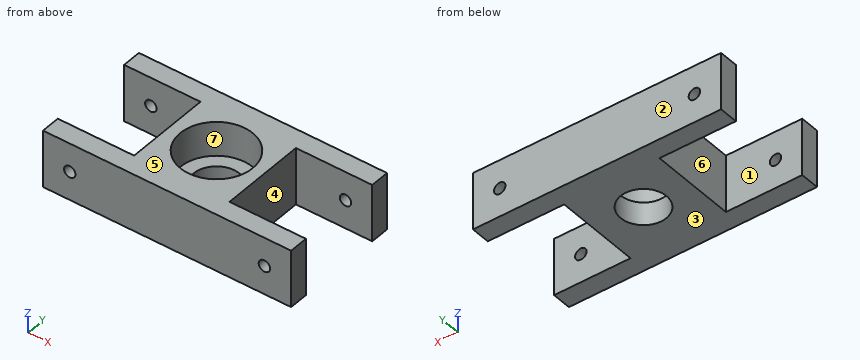
Autodesk Inventor part; units mm, degrees
ref_plane "YZ Plane" through (0, 0, 0) normal (1, 0, 0) x (0, 1, 0)
ref_plane "XZ Plane" through (0, 0, 0) normal (0, 1, 0) x (-1, 0, 0)
ref_plane "XY Plane" through (0, 0, 0) normal (0, 0, 1) x (1, 0, 0)
sketch "Boceto1" plane through (0, 0, 0) normal (0, 0, 1) x (1, 0, 0)
  line L0 (-12.5, 16.25) -> (12.5, 16.25)
  line L1 (12.5, 16.25) -> (12.5, -16.25)
  line L2 (12.5, -16.25) -> (-12.5, -16.25)
  line L3 (-12.5, -16.25) -> (-12.5, 16.25)
  line L4 (-12.5, 16.25) -> (12.5, -16.25) construction
  line L5 (12.5, 16.25) -> (-12.5, -16.25) construction
  point P0 (0, 0)
  dimension "d0" = 25
  dimension "d1" = 32.5
extrude "Extrusión1" add sketch "Boceto1" against normal blind 15
sketch "Boceto4" plane through (0, 0, 0) normal (0, 0, 1) x (1, 0, 0)
  circle A0 centre (0, 0.5) radius 9.5
  line L0 (-12.5, -16.25) -> (12.5, -16.25)
  line L1 (0, 0) -> (0, 22.8152) construction
  dimension "d20" = 19
  dimension "d21" = 16.75
extrude "Extrusión4" cut sketch "Boceto4" against normal blind 9
sketch "Boceto5" plane through (0, 0.5, -9) normal (0, 0, 1) x (1, 0, 0)
  circle A0 centre (0, 0) radius 6
  circle A1 centre (0, 0) radius 9.5
  point P0 (0, -0.5)
  point P1 (-7.5, -5.831)
  point P2 (7.5, -5.831)
  dimension "d27" = 12
extrude "Extrusión5" cut sketch "Boceto5" against normal through all contours A0
sketch "Boceto6" plane through (0, 0, -15) normal (0, 0, -1) x (-1, 0, 0)
  line L0 (-12.5, 16.25) -> (-32.5, 16.25)
  line L1 (-32.5, 16.25) -> (-32.5, 11.25)
  line L2 (-32.5, 11.25) -> (-12.5, 11.25)
  line L3 (-12.5, 11.25) -> (-12.5, 16.25)
  line L4 (4.8011, 9.4889) -> (4.8011, -13.0562) construction
  line L5 (0, 15.379) -> (0, -16.25) construction
  line L6 (-12.5, -16.25) -> (12.5, -16.25)
  line L7 (12.5, -16.25) -> (12.5, 16.25) construction
  line L8 (12.5, 0) -> (-12.5, 0) construction
  line L9 (-12.5, 16.25) -> (-12.5, -16.25) construction
  line L10 (-12.5, -16.25) -> (-32.5, -16.25)
  line L11 (-32.5, -16.25) -> (-32.5, -11.25)
  line L12 (-32.5, -11.25) -> (-12.5, -11.25)
  line L13 (-12.5, -11.25) -> (-12.5, -16.25)
  line L14 (12.5, 16.25) -> (32.5, 16.25)
  line L15 (32.5, 16.25) -> (32.5, 11.25)
  line L16 (32.5, 11.25) -> (12.5, 11.25)
  line L17 (12.5, 11.25) -> (12.5, 16.25)
  line L18 (12.5, 16.25) -> (12.5, -16.25) construction
  line L19 (12.5, -16.25) -> (32.5, -16.25)
  line L20 (12.5, -11.25) -> (12.5, -16.25)
  line L21 (32.5, -11.25) -> (12.5, -11.25)
  line L22 (32.5, -16.25) -> (32.5, -11.25)
  point P0 (0, 0)
  dimension "d30" = 5
  dimension "d31" = 20
extrude "Extrusión6" add sketch "Boceto6" against normal up to surface (15 mm away)
sketch "Boceto8" plane through (-32.5, 16.25, 0) normal (0, 1, 0) x (1, 0, 0)
  line L0 (0, 15) -> (0, 0) construction
  line L1 (0, 7.5) -> (65, 7.5) construction
  line L2 (65, 15) -> (65, 0) construction
  circle A0 centre (7, 7.5) radius 1.5
  circle A1 centre (58, 7.5) radius 1.5
  line L3 (65, 0) -> (0, 0)
  point P0 (32.5, 0)
  point P1 (32.5, 0)
  dimension "d43" = 3
  dimension "d44" = 3
  dimension "d45" = 51
  dimension "d46" = 25.5
extrude "Extrusión8" cut sketch "Boceto8" against normal through all
sketch "Boceto10" plane through (-32.5, 16.25, 0) normal (0, 1, 0) x (1, 0, 0)
  point P0 (32.5, 0)
properties part number "soporte_eje_omni_3DPrint"
Input: part model. Units: mm. Frame: model coordinates. Face numbers are marked on the shaded views. A direction names the side the tool comes from. Coordinates: 2 decimals unless noted, no trailing zeros. Order: outer loops, then holes, each group sorted by start corner. A loop starts at its lowest first (then second) coordinate and runs counter-clockwise, first axis right, second up.
1. Cut plane D-D, the plane z = -13. Return loops of the section in (x, y), plus the area to 3 significant figures.
Checked values:
outline: (-32.5, -16.25) - (32.5, -16.25) - (32.5, -11.25) - (12.5, -11.25) - (12.5, 11.25) - (32.5, 11.25) - (32.5, 16.25) - (-32.5, 16.25) - (-32.5, 11.25) - (-12.5, 11.25) - (-12.5, -11.25) - (-32.5, -11.25) - close; hole circle Ø12 at (0, 0.5)
area: 1,100 mm2
2. Contact query for flat-ended pins moving along their axis: P1, Ø11.5, axis at x = 0, y = 0.5, coming from the +Z side; P2, Ø1.5, axis at y = 3.5, z = -11.5, coming from the -X side; P3, Ø6, axis at y = 5, z = -6.5, coming from the +X side. Output: stop coordinate, or through.
Checked values:
P1: passes through
P2: stops at x = -12.5
P3: stops at x = 12.5
3. Cut plane A-A, the plane z = -7.5. Count the separate pieces of the cut face and the enclosed holes in it, plus the area to 3 significant figures.
Checked values:
separate pieces: 5
enclosed holes: 1
area: 869 mm2
4. Access query for the marked faces 4, 5, 6 and 7. Directions: +Z, -Z, +X, -X, +Y, -Y. A direction counts if a zero-diameter tool reaches every point of the face in a straight line with its end or side. Return the directions, or none.
Checked values:
face 4: +Z, -Z, +X
face 5: +Z, +X, -X, +Y, -Y
face 6: +Z, -Z, -X
face 7: +Z
5. Cut plane B-B, the plane x = 0. Return loops of the section in (y, z).
Checked values:
outline: (-16.25, -15) - (-5.5, -15) - (-5.5, -9) - (-9, -9) - (-9, 0) - (-16.25, 0) - close; (6.5, -15) - (16.25, -15) - (16.25, 0) - (10, 0) - (10, -9) - (6.5, -9) - close
6. Draft query along Y for the marked faces 1, 2 and 3. Return one class per face: +Y half, -Y half, draft (parallel to the pull), parting line (faces both ways), or undercut.
Checked values:
face 1: undercut
face 2: +Y half
face 3: draft
7. Ray query, line 1 along X through (y, z) = (14.75, -7.5); line 2 along Y through (x, z) = (-18, -12.25); line 3 along Y through (x, z) = (0, -6.75). Return the intervals inside material, ascending.
Checked values:
line 1: x = -32.5 to -27, -24 to 24, 27 to 32.5
line 2: y = -16.25 to -11.25, 11.25 to 16.25
line 3: y = -16.25 to -9, 10 to 16.25
8. Cut plane C-C, the plane x = 25.5. Return loops of the section in (y, z).
Checked values:
outline: (-16.25, -15) - (-11.25, -15) - (-11.25, -9) - (-16.25, -9) - close; (-16.25, -6) - (-11.25, -6) - (-11.25, 0) - (-16.25, 0) - close; (11.25, -15) - (16.25, -15) - (16.25, -9) - (11.25, -9) - close; (11.25, -6) - (16.25, -6) - (16.25, 0) - (11.25, 0) - close
